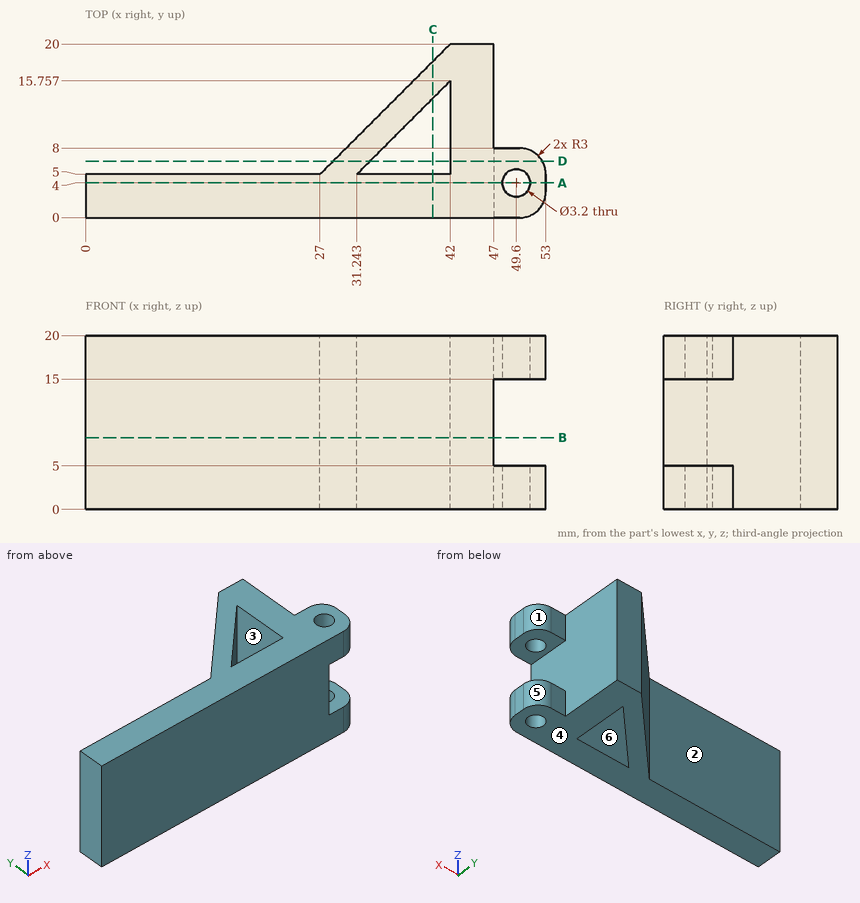
Input: dimensioned drawing with shaded views. Units: mm. Origin: part minimum x, y, z. A direction names the side the tool comes from. Give positions to 0.01 mm unless a question says otherwise; leave off trailing zeros. Write each loop counter-clockwise with the first axis right and the second up, starting at its lowest first coordinate (ties: lowest second). Pieces come first, ordered by that corner, then holes.
1. Draft query along Y for the marked faces 3, 4, 5 and 6. Return one class per face: released by +Y, released by -Y, zero draft, split by the parting line, or undercut.
2. Section query B-B, the plane z = 8.25. Return loops of the section in (x, y).
3. Section query D-D, the plane y = 6.5. Return loops of the section in (x, z), then the cut area to 3 significant figures.
4. Reachability of the marked faces 1 and 2 from +Z, -Z, +X, -X, +Y, -Y: full face, straight path, thin tool, end or side. Return the list, or none.
5. Section query C-C, the plane x = 40. Return loops of the section in (y, z), then the cut area to 3 significant figures.
6. Section query A-A, the plane y = 4. Return loops of the section in (x, z).
7. Pin query (flat end, axial travel): P1, Ø4, axis at x = 49.6, y = 4, coming from the -Z side; P2, Ø3, axis at x = 36.5, z = 9, coming from the +Y side; P3, Ø0.9, axis at x = 49, z = 2.5, coming from the +Y side; P4, Ø10, axis at x = 20, z = 6.5, coming from the +Y side. Return the tip coordinate at first contact, or that it passes through.
8. Line query: probe 1 along X at (y, z) = (4, 17.55); probe 2 along Y at (x, z) = (49.6, 17.1); probe 3 along Y at (x, z) = (9, 14). Output: solid intervals per line, ascending.
Computed:
1. face 3: undercut
1. face 4: zero draft
1. face 5: released by +Y
1. face 6: undercut
2. outline: (0, 0) - (47, 0) - (47, 20) - (42, 20) - (27, 5) - (0, 5) - close; hole (31.24, 5) - (42, 5) - (42, 15.76) - close
3. outline: (28.5, 0) - (32.74, 0) - (32.74, 20) - (28.5, 20) - close; (42, 0) - (52.6, 0) - (52.6, 5) - (47, 5) - (47, 15) - (52.6, 15) - (52.6, 20) - (42, 20) - close
3. area: 241 mm2
4. face 1: +Z, -Z, +X, +Y
4. face 2: +Z, -Z, -X, +Y
5. outline: (0, 0) - (5, 0) - (5, 20) - (0, 20) - close; (13.76, 0) - (18, 0) - (18, 20) - (13.76, 20) - close
5. area: 185 mm2
6. outline: (0, 0) - (48, 0) - (48, 5) - (47, 5) - (47, 15) - (48, 15) - (48, 20) - (0, 20) - close; (51.2, 0) - (53, 0) - (53, 5) - (51.2, 5) - close; (51.2, 15) - (53, 15) - (53, 20) - (51.2, 20) - close
7. P1: stops at z = 0
7. P2: stops at y = 16
7. P3: stops at y = 8
7. P4: stops at y = 5
8. probe 1: x = 0 to 48, 51.2 to 53
8. probe 2: y = 0 to 2.4, 5.6 to 8
8. probe 3: y = 0 to 5
